The listing builds one solid part. Answer for the finished solid, in the listing's coordinates (mm). Round coordinates to 2 decimals unless told otherwise and drop trailing zeros. Write each loop counter-clockwise with the first axis right and the second up, starting at its lowest first coordinate (ties: lowest second). Pieces come first, ordered by that corner, then holes. Notation, with made-up numbers: (54.25, 6) - (66.25, 6) arc R22 ccw to (66.25, 26) - close; hole circle Ø7 at (52.5, 42.25). An arc over 180 degrees is marked (long way). Use a Markdown table: item, result. Add a question column.
1) Find the intervals of material crossed by probe 1 along Z at (x, y) = (75, 107.5); probe 2 along X at (y, z) = (66, 0); probe 3 along X at (y, z) = (90, 0), in increasing order. Write a range as from..to.
2) A cutting plane is placed at C-C (x = -433). Give the vertices of the cut face in (y, z), then the cut area to 3 significant figures.
3) A cutting plane is placed at A-A (x = -936). Give the vertices of the cut face in (y, z), then the cut area to 3 significant figures.
4) Each of these flat-tipped pins is pushed along its axis until it touches: P1, Ø4, axis at x = -573.5, y = 906, coming from the -Z side; P2, Ø6, axis at y = 616.5, z = 27.5, coming from the -X side; P3, Ø5, axis at x = -426.5, z = -43.5, coming from the -Y side. Where does it stop, or does it pass through?
5) A cutting plane is placed at B-B (y = 1020.5). Give the vertices of the cut face in (x, z).
6) A cutting plane is placed at D-D (y = 1429.5). Give the vertices of the cut face in (x, z), then the cut area to 3 significant figures.
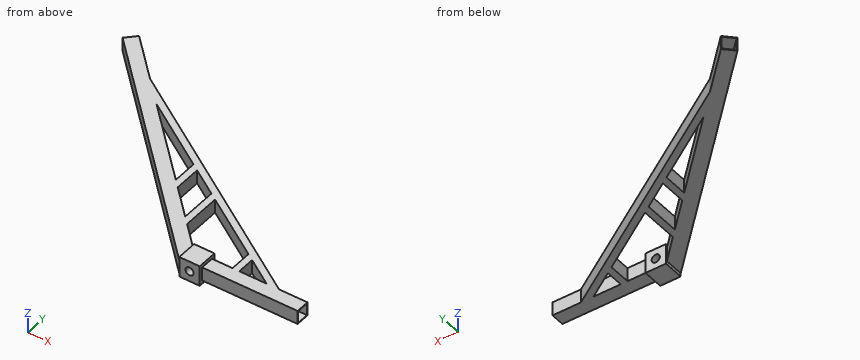
Autodesk Inventor part; units mm, degrees
ref_plane "YZ Plane" through (0, 0, 0) normal (1, 0, 0) x (0, 1, 0)
ref_plane "XZ Plane" through (0, 0, 0) normal (0, 1, 0) x (-1, 0, 0)
ref_plane "XY Plane" through (0, 0, 0) normal (0, 0, 1) x (1, 0, 0)
sketch "Sketch1" plane through (0, 0, 0) normal (0, 0, 1) x (1, 0, 0)
  line L0 (0, 0) -> (150, 0)
  line L1 (150, 0) -> (150, 150)
  line L2 (150, 150) -> (0, 150)
  line L3 (0, 150) -> (0, 0)
  line L4 (0, 0) -> (-1500, 1500)
  line L5 (-1500, 1500) -> (-1429.2893, 1570.7107)
  line L6 (-1429.2893, 1570.7107) -> (0, 141.4214)
  line L7 (0, 141.4214) -> (0, 0)
  line L8 (150, 100) -> (150, 0)
  line L9 (150, 0) -> (150, 125)
  line L10 (150, 125) -> (850, 125)
  line L11 (850, 125) -> (850, 25)
  line L12 (850, 25) -> (150, 25)
  line L13 (150, 25) -> (150, 125)
  dimension "d0" = 150
  dimension "d1" = 150
  dimension "d8" = 1500
  dimension "d9" = 100
  dimension "d12" = 125
  dimension "d13" = 700
  dimension "d14" = 100
extrude "Extrusion3" add sketch "Sketch1" along normal mid plane 150 contours L3 L2 L1 L0
sketch "Sketch3" plane through (0, 0, 0) normal (0, 0, 1) x (1, 0, 0)
  line L0 (0, 0) -> (-1500, 1500)
  line L1 (0, 0) -> (2121.3203, 0) construction
  line L2 (-1500, 1500) -> (-1429.2893, 1570.7107)
  line L3 (-1429.2893, 1570.7107) -> (0, 141.4214)
  line L4 (0, 0) -> (0, 141.4214)
  line L5 (150, 0) -> (150, 125)
  line L6 (150, 125) -> (850, 125)
  line L7 (850, 125) -> (850, 25)
  line L8 (850, 25) -> (150, 25)
  line L9 (150, 25) -> (150, 125)
  dimension "d17" = 135
  dimension "d18" = 1500
  dimension "d19" = 100
  dimension "d20" = 125
  dimension "d21" = 700
  dimension "d22" = 100
extrude "Extrusion4" add sketch "Sketch3" along normal mid plane 100
sketch "Sketch4" plane through (-1500, 1500, -50) normal (-0.7071, 0.7071, 0) x (-0.7071, -0.7071, 0)
  line L0 (-95, 95) -> (-5, 95)
  line L1 (-5, 95) -> (-5, 5)
  line L2 (-5, 5) -> (-95, 5)
  line L3 (-95, 5) -> (-95, 95)
  line L4 (-95, 95) -> (-5, 5) construction
  line L5 (-5, 95) -> (-95, 5) construction
  point P0 (0, 50)
  point P1 (-50, 50)
  dimension "d25" = 90
  dimension "d26" = 90
extrude "Extrusion5" cut sketch "Sketch4" against normal blind 2122.5
sketch "Sketch5" plane through (0, 0, 0) normal (0, 0, 1) x (1, 0, 0)
  line L0 (0, 132.8216) -> (69.0672, 132.8216)
  line L1 (69.0672, 132.8216) -> (69.0672, 2.6564)
  line L2 (69.0672, 2.6564) -> (0, 2.6564)
  line L3 (0, 2.6564) -> (0, 132.8216)
  point P0 (0, 0)
extrude "Extrusion6" add sketch "Sketch5" along normal mid plane 100.5
sketch "Sketch6" plane through (0, 0, 0) normal (0, 0, 1) x (1, 0, 0)
  point P0 (0, 0)
sketch "Sketch7" plane through (0, 150, 75) normal (0, 1, 0) x (1, 0, 0)
  circle A0 centre (75, 75) radius 30
  point P0 (0, 75)
  dimension "d31" = 60
extrude "Extrusion7" cut sketch "Sketch7" against normal blind 340
sketch "Sketch8" plane through (850, 25, 50) normal (1, 0, 0) x (0, 0, -1)
  line L0 (5, 95) -> (95, 95)
  line L1 (95, 95) -> (95, 5)
  line L2 (95, 5) -> (5, 5)
  line L3 (5, 5) -> (5, 95)
  line L4 (5, 95) -> (95, 5) construction
  line L5 (95, 95) -> (5, 5) construction
  point P0 (50, -25)
  point P1 (50, 50)
  dimension "d34" = 90
  dimension "d35" = 90
extrude "Extrusion8" cut sketch "Sketch8" against normal blind 700
sketch "Sketch9" plane through (0, 0, 0) normal (0, 0, 1) x (1, 0, 0)
  point P0 (0, 0)
sketch "Sketch10" plane through (0, 0, 0) normal (0, 0, 1) x (1, 0, 0)
  line L0 (150, 125) -> (550, 125)
  line L1 (550, 125) -> (-971.9923, 1113.3934)
  line L2 (550, 125) -> (2376.4621, 125) construction
  line L3 (550, 125) -> (641.8039, 125)
  line L4 (641.8039, 125) -> (-1142.0421, 1283.4431)
  line L5 (-971.9923, 1113.3934) -> (-1142.0421, 1283.4431)
  line L6 (-971.9923, 1113.3934) -> (-731.5056, 1113.3934) construction
  line L7 (150, 125) -> (300, 125)
  point P0 (0, 0)
  dimension "d41" = 147
  dimension "d42" = 50
  dimension "d43" = 400
  dimension "d44" = 135
  dimension "d45" = 150
extrude "Extrusion9" add sketch "Sketch10" along normal mid plane 100
sketch "Sketch11" plane through (0, 0, 50) normal (0, 0, 1) x (1, 0, 0)
  line L0 (0, 141.4214) -> (-971.9344, 1113.3558)
  line L1 (-971.9344, 1113.3558) -> (550, 125)
  line L2 (550, 125) -> (150, 125)
  line L3 (150, 125) -> (300, 125)
  line L4 (300, 125) -> (300, 287.3519)
  line L5 (300, 125) -> (350, 125)
  line L6 (350, 125) -> (350, 254.8815)
  line L7 (300, 287.3519) -> (350, 254.8815)
  line L8 (305, 130) -> (305, 278.143)
  line L9 (0, 141.4214) -> (-212.132, 353.5534)
  line L10 (-212.132, 353.5534) -> (-247.4874, 388.9087)
  line L11 (-93.5014, 542.8947) -> (-50.6311, 515.0544)
  line L12 (0, 141.4214) -> (-459.6194, 601.0408)
  line L13 (-459.6194, 601.0408) -> (-494.9747, 636.3961)
  line L14 (-212.132, 353.5534) -> (-212.132, 619.9343)
  line L15 (-162.132, 303.5534) -> (-162.132, 587.464)
  line L16 (-212.132, 353.5534) -> (-175.196, 316.6173)
  line L17 (-212.132, 619.9343) -> (-162.132, 587.464)
  line L18 (-459.6194, 601.0408) -> (-459.6194, 780.6545)
  line L19 (-409.6194, 748.1841) -> (-409.6194, 551.0408)
  line L20 (-409.6194, 551.0408) -> (-459.6194, 601.0408)
  line L21 (-409.6194, 551.0408) -> (-459.6194, 601.0408)
  line L22 (-459.6194, 601.0408) -> (-409.6194, 551.0408)
  line L23 (-459.6194, 780.6545) -> (-409.6194, 748.1841)
  dimension "d48" = 150
  dimension "d49" = 50
  dimension "d51" = 300
  dimension "d52" = 50
  dimension "d54" = 650
  dimension "d55" = 50
  dimension "d71" = 50
  dimension "d72" = 50
sketch "Sketch13" plane through (0, 0, 50) normal (0, 0, 1) x (1, 0, 0)
  line L0 (-314.5783, 746.0819) -> (-298.0455, 762.6147)
  line L1 (-333.4008, 797.97) -> (-298.0455, 762.6147)
  line L2 (-357.4486, 773.9222) -> (-333.4008, 797.97)
  line L3 (-971.9344, 1113.3558) -> (550, 125)
  line L4 (-314.5783, 746.0819) -> (-357.4486, 773.9222)
  line L5 (-333.4008, 797.97) -> (-298.0455, 762.6147)
  line L6 (-298.0455, 762.6147) -> (-314.5783, 746.0819)
  line L7 (-333.4008, 797.97) -> (-357.4486, 773.9222)
  point P0 (-393.5938, 737.777)
extrude "Extrusion11" cut sketch "Sketch13" against normal blind 228.5
sketch "Sketch16" plane through (0, 0, 0) normal (0, 0, 1) x (1, 0, 0)
  point P0 (0, 0)
extrude "Extrusion13" add sketch "Sketch11" against normal blind 100 contours L1 L6 L2 L4 | L0 L14 L1 L15 | L19 L0 L18 L1
properties part number "kepala baru" material "Steel, Mild"
Entries:
| question | item | result |
|---|---|---|
| 1 | probe 1 | z = -75..-30, 30..75 |
| 1 | probe 2 | x = -66..-58.93, 0..45, 105..150 |
| 1 | probe 3 | x = -90..-82.93, 0..45, 105..150 |
| 2 | outline | (433, -50) - (822.99, -50) - (822.99, 50) - (433, 50) - close; hole (440.07, -45) - (567.35, -45) - (567.35, 45) - (440.07, 45) - close |
| 2 | area | 27,500 mm² |
| 3 | outline | (936, -50) - (1077.42, -50) - (1077.42, 50) - (936, 50) - close; (1090.02, -50) - (1149.64, -50) - (1149.64, 50) - (1090.02, 50) - close; hole (943.07, -45) - (1070.35, -45) - (1070.35, 45) - (943.07, 45) - close |
| 3 | area | 8,650 mm² |
| 4 | P1 | stops at z = -50 |
| 4 | P2 | stops at x = -619.5 |
| 4 | P3 | stops at y = 424 |
| 5 | outline | (-1020.5, -50) - (-879.08, -50) - (-879.08, 50) - (-1020.5, 50) - close; (-828.95, -50) - (-737.15, -50) - (-737.15, 50) - (-828.95, 50) - close; hole (-1013.43, -45) - (-886.15, -45) - (-886.15, 45) - (-1013.43, 45) - close |
| 6 | outline | (-1429.5, -50) - (-1288.08, -50) - (-1288.08, 50) - (-1429.5, 50) - close; hole (-1422.43, -45) - (-1295.15, -45) - (-1295.15, 45) - (-1422.43, 45) - close |
| 6 | area | 2,690 mm² |
